```python
from build123d import *

# Parameters (mm, degrees)
F0_R     = 5
F0_R_2   = 4
F1_DEPTH = 15


with BuildPart() as f1:
    # F0 (on Top) → F1 (new body)
    with BuildSketch(Plane.XY):
        with BuildLine():
            Line((15.090626, 16.689009), (-21.443711, 49.724285))
            ThreePointArc((-21.443711, 49.724285), (-49.611346, 49.382679), (-49.497475, 21.213203))
            Line((-49.497475, 21.213203), (-45.750738, 18.269213))
            Line((-45.750738, 18.269213), (-22.5, 0))
            Line((-22.5, 0), (-22.5, -85))
            ThreePointArc((-22.5, -85), (0, -107.5), (22.5, -85))
            Line((22.5, -85), (22.5, 0))
            ThreePointArc((22.5, 0), (20.5644, 9.129921), (15.090626, 16.689009))
        make_face()
        with Locations((0, -85)):
            Circle(F0_R, mode=Mode.SUBTRACT)
        with Locations((-35.355339, 35.355339)):
            Circle(F0_R_2, mode=Mode.SUBTRACT)
        Circle(F0_R_2, mode=Mode.SUBTRACT)
    extrude(amount=F1_DEPTH)


solid = f1.part
```
Model file for the job. Use its own axes, mm. A direction names the side the tool comes from. Give positions to 0.01 mm unless a question says otherwise; leave off trailing zeros. Loops run counter-clockwise (first coordinate to the right, second up) from the corner with the lowest first, then second, coordinate; pieces in that order, holes last. Notation, with made-up numbers: (45.5, 63) -> (71.5, 63) arc R22 ccw to (71.5, 91) -> close; hole circle Ø7 at (56, 51). An arc over 180 degrees is marked (long way). Use CSV: the item, a comma, the result in double quotes. Start each with the question number.
1) Slice it at C-C on y = -49. Give the cut face in (x, z).
2) Slice it at A-A on x = 0. Give the cut face in (y, z), plus the area to 3 significant figures.
3) Flat gauge pins, fed straight in: pin 1 Ø1.5 at (x, z) = (10, 12) entering from -Y; pin 2 Ø5 at (y, z) = (-55, 7.5) entering from -X; pin 3 Ø3 at (x, z) = (14, 8) entering from +Y. Where does each tip first touch, or does it go through?
4) Mould opens along X. For faces 3 (the cylindrical face through (-0.495, -107.495, 7.395)), 4 (the flat face through (-8, -25, 15)), 5 (the cylindrical face through (-1.08, -89.88, 7.4)), 6 (the cylindrical face through (-31.54, 36.56, 7.4)) say: released by +X, released by -X, zero draft, split by the parting line, or undercut.
5) Slice it at B-B on z = 11.5. Give the cut face in (x, y), plus the area to 3 significant figures.
6) Tool access for faces 1 (the flat face through (-22.5, -42, 7)), 2 (the cylindrical face through (-0.867, -3.905, 7.395)): list every direction of +Z, -Z, +X, -X, +Y, -Y with a clear straight run to the whole face (end or side of a thin tool).
7) Wall check: line 1 (Y direction, x = 0, z = 11.5); line 2 (Y direction, x = 3, z = 4.75); line 3 (X direction, y = -67.5, z = 8.25). Give the ranges that are in metal, low to high.
8) Slice it at D-D on x = -17. Give the cut face in (y, z).
Computed values:
1,outline,"(-22.5, 0) -> (22.5, 0) -> (22.5, 15) -> (-22.5, 15) -> close"
2,outline,"(-107.5, 0) -> (-90, 0) -> (-90, 15) -> (-107.5, 15) -> close; (-80, 0) -> (-4, 0) -> (-4, 15) -> (-80, 15) -> close; (4, 0) -> (30.33, 0) -> (30.33, 15) -> (4, 15) -> close"
2,area,"1,800 mm^2"
3,pin 1,"stops at y = -105.51"
3,pin 2,"stops at x = -22.5"
3,pin 3,"stops at y = 19.03"
4,face 3,"split by the parting line"
4,face 4,"zero draft"
4,face 5,"undercut"
4,face 6,"undercut"
5,outline,"(-49.5, 21.21) -> (-22.5, 0) -> (-22.5, -85) arc R22.5 ccw to (22.5, -85) -> (22.5, 0) arc R22.5 ccw to (15.09, 16.69) -> (-21.44, 49.72) arc R20 ccw to start; hole circle Ø8 at (-35.36, 35.36); hole circle Ø10 at (0, -85); hole circle Ø8 at (0, 0)"
5,area,"7,070 mm^2"
6,face 1,"+Z, -Z, -X, -Y"
6,face 2,"+Z, -Z"
7,line 1,"y = -107.5 to -90, -80 to -4, 4 to 30.33"
7,line 2,"y = -107.3 to -89, -81 to -2.65, 2.65 to 27.62"
7,line 3,"x = -22.5 to 22.5"
8,outline,"(-99.74, 0) -> (45.71, 0) -> (45.71, 15) -> (-99.74, 15) -> close"
